from build123d import *

# Parameters (mm, degrees)
SKETCH6_R           = 5.461
BOSS_EXTRUDE4_DEPTH = 15.24
SKETCH7_OUTSIDE_W   = 17.262
SKETCH7_OUTSIDE_H   = 17.262
SKETCH7_OUTSIDE_R   = 2.921
CUT_EXTRUDE2_DEPTH  = 8.89
SKETCH8_R           = 4.8895
CUT_EXTRUDE3_DEPTH  = 5.08
FILLET2_R           = 1.27


with BuildPart() as part:
    # Sketch6 → Boss-Extrude4 (new body)
    with BuildSketch(Plane(origin=(0, 0, 0), x_dir=(1, 0, 0), z_dir=(0, 1, 0))):
        with Locations(Location((0, 0, 0), (0, 0, 90))):
            Circle(SKETCH6_R)
    extrude(amount=BOSS_EXTRUDE4_DEPTH)

    # Sketch7 outside → Cut-Extrude2 (cut)
    with BuildSketch(Plane(origin=(0, 15.24, 0), x_dir=(1, 0, 0), z_dir=(0, 1, 0))):
        Rectangle(SKETCH7_OUTSIDE_W, SKETCH7_OUTSIDE_H)
        with Locations(Location((0, 0, 0), (0, 0, 270))):
            Circle(SKETCH7_OUTSIDE_R, mode=Mode.SUBTRACT)
    extrude(amount=-CUT_EXTRUDE2_DEPTH, mode=Mode.SUBTRACT)

    # Sketch8 → Cut-Extrude3 (cut)
    with BuildSketch(Plane.XZ):
        with Locations(Location((0, 0, 0), (0, 0, 270))):
            Circle(SKETCH8_R)
    extrude(amount=-CUT_EXTRUDE3_DEPTH, mode=Mode.SUBTRACT)

    # Fillet2
    fillet2_edges = [part.edges().sort_by_distance(p)[0] for p in [
        (0, 6.35, -2.921),
    ]]
    fillet(fillet2_edges, radius=FILLET2_R)


solid = part.part
Could you check a few things on this model? Use its own coordinates, in mm. A direction names the side the tool comes from. Coordinates: 2 decimals unless noted, no trailing zeros. Order: outer loops, then holes, each group sorted by start corner. A loop starts at its lowest first (then second) coordinate and runs counter-clockwise, first axis right, second up.
Q1. Please list where these lines run through material, in increasing order: L1, parallel to X at y = 2.7, z = 0; L2, parallel to Y at x = -3.5, z = -2.5; L3, parallel to Z at x = 2.5, y = 1.
Q2. Which directions (+Z, -Z, +X, -X, +Y, -Y) give clear straight access to the entire face, cutting with the end or side of a thin tool? Please do faces 4 (the flat face through (0, 15.24, 0)), 5 (the cylindrical face through (-4.773, 2.504, 1.06)), 6 (the flat face through (2, 6.35, 4)).
Q3. Suppose I cut it at A-A on x = 0. Please give me the cut outline in (y, z), and give its area (3 significant figures).
Q4. Suppose I cut it at D-D on y = 10.5. Please give me the cut outline in (x, z), and give its area (3 significant figures).
Q5. Suppose I cut it at C-C on z = 0. Please give me the cut outline in (x, y).
Q6. Suppose I cut it at B-B on y = 1. Please give me the cut outline in (x, z), and give its area (3 significant figures).
Q7. Thinking about a two-plate mould opening in X: for faces 1 (the cylindrical face through (2.092, 3.131, -5.045)), 2 (the flat face through (5, 0, 1)), 3 (the flat face through (0, 5.08, 0)), which applies, released by +X, released by -X, zero draft, split by the parting line, or undercut?
Q8. Will these pins go through, and if not, where does the flat tip stop? pin 1 (5 mm diameter, centred on y = 13.5, z = 2.5, fed in from -X); pin 2 (5 mm diameter, centred on y = 8.5, z = -1, fed in from +X); pin 3 (1 mm diameter, centred on x = -2.5, y = 5, fed in from +Z); pin 4 (1.5 mm diameter, centred on y = 12.5, z = 2, fed in from +X).
Answer:
1. L1: x = -5.46 to -4.89, 4.89 to 5.46
1. L2: y = 5.08 to 6.35
1. L3: z = -4.86 to -4.2, 4.2 to 4.86
2. face 4: +Z, -Z, +X, -X, +Y
2. face 5: -Y
2. face 6: +Y
3. outline: (0, -5.46) - (6.35, -5.46) - (6.35, -4.19) arc R1.27 cw to (7.62, -2.92) - (15.24, -2.92) - (15.24, 2.92) - (7.62, 2.92) arc R1.27 cw to (6.35, 4.19) - (6.35, 5.46) - (0, 5.46) - (0, 4.89) - (5.08, 4.89) - (5.08, -4.89) - (0, -4.89) - close
3. area: 72.3 mm2
4. outline: circle Ø5.84 at (0, 0)
4. area: 26.8 mm2
5. outline: (-5.46, 0) - (-4.89, 0) - (-4.89, 5.08) - (4.89, 5.08) - (4.89, 0) - (5.46, 0) - (5.46, 6.35) - (4.19, 6.35) arc R1.27 cw to (2.92, 7.62) - (2.92, 15.24) - (-2.92, 15.24) - (-2.92, 7.62) arc R1.27 cw to (-4.19, 6.35) - (-5.46, 6.35) - close
6. outline: circle Ø10.92 at (0, 0); hole circle Ø9.78 at (0, 0)
6. area: 18.6 mm2
7. face 1: split by the parting line
7. face 2: zero draft
7. face 3: undercut
8. pin 1: stops at x = -2.92
8. pin 2: stops at x = 5.46
8. pin 3: stops at z = 5.08
8. pin 4: stops at x = 2.64
